```python
from build123d import *

# Parameters (mm, degrees)
SKETCH1_R           = 1.8
SKETCH1_W           = 13
SKETCH1_H           = 7.25
BOSS_EXTRUDE1_DEPTH = 1
SKETCH2_R           = 3
SKETCH2_R_2         = 1.8
BOSS_EXTRUDE2_DEPTH = 5.8
FILLET4_R           = 2
FILLET5_R           = 2
FILLET6_R           = 2
FILLET7_R           = 2


with BuildPart() as part:
    # Sketch1 → Boss-Extrude1 (new body)
    with BuildSketch(Plane.XY):
        with BuildLine():
            Line((-6.5, 11), (6.5, 11))
            Line((6.5, 11), (10.25, 11))
            Line((10.25, 11), (10.25, 3))
            ThreePointArc((10.25, 3), (13.25, 0), (10.25, -3))
            Line((10.25, -3), (10.25, -11))
            Line((10.25, -11), (6.5, -11))
            Line((6.5, -11), (-6.5, -11))
            Line((-6.5, -11), (-10.25, -11))
            Line((-10.25, -11), (-10.25, -3))
            ThreePointArc((-10.25, -3), (-13.25, 0), (-10.25, 3))
            Line((-10.25, 3), (-10.25, 11))
            Line((-10.25, 11), (-6.5, 11))
        make_face()
        with Locations(Location((-10.25, 0, 0), (0, 0, 180))):
            Circle(SKETCH1_R, mode=Mode.SUBTRACT)
        with Locations((10.25, 0)):
            Circle(SKETCH1_R, mode=Mode.SUBTRACT)
        with Locations((0, -4.875)):
            Rectangle(SKETCH1_W, SKETCH1_H, mode=Mode.SUBTRACT)
        with Locations((0, 4.875)):
            Rectangle(SKETCH1_W, SKETCH1_H, mode=Mode.SUBTRACT)
    extrude(amount=BOSS_EXTRUDE1_DEPTH)

    # Sketch2 → Boss-Extrude2 (add)
    with BuildSketch(Plane.XY.offset(1)):
        with Locations(Location((-10.25, 0, 0), (0, 0, 270))):
            Circle(SKETCH2_R)
        with Locations(Location((-10.25, 0, 0), (0, 0, 180))):
            Circle(SKETCH2_R_2, mode=Mode.SUBTRACT)
        with Locations(Location((10.25, 0, 0), (0, 0, 180))):
            Circle(SKETCH2_R)
        with Locations(Location((10.25, 0, 0), (0, 0, 180))):
            Circle(SKETCH2_R_2, mode=Mode.SUBTRACT)
    extrude(amount=BOSS_EXTRUDE2_DEPTH)

    # Fillet4
    fillet4_edges = [part.edges().sort_by_distance(p)[0] for p in [
        (-10.25, 11, 0.5),
    ]]
    fillet(fillet4_edges, radius=FILLET4_R)

    # Fillet5
    fillet5_edges = [part.edges().sort_by_distance(p)[0] for p in [
        (10.25, 11, 0.5),
    ]]
    fillet(fillet5_edges, radius=FILLET5_R)

    # Fillet6
    fillet6_edges = [part.edges().sort_by_distance(p)[0] for p in [
        (-10.25, -11, 0.5),
    ]]
    fillet(fillet6_edges, radius=FILLET6_R)

    # Fillet7
    fillet7_edges = [part.edges().sort_by_distance(p)[0] for p in [
        (10.25, -11, 0.5),
    ]]
    fillet(fillet7_edges, radius=FILLET7_R)


solid = part.part
```
Can you work these out from the model? Positions are in its coordinate system, mm. A direction names the side the tool comes from. Give positions to 0.01 mm unless a question says otherwise; leave off trailing zeros. Loops run counter-clockwise (first coordinate to the right, second up) from the corner with the lowest first, then second, coordinate; pieces in that order, holes last. Notation, with made-up numbers: M -30,-18.75 L 0,-18.75 A21 ccw 0,0.25 Z; hole C 46,-3.75 d3. An arc over 180 degrees is marked long. Answer in a Markdown table with one row per item.
1. Suppose I cut it at B-B on x = -5.25. Write out the boundary of the cut face in (y, z).
Taken from the geometry:
| item | result |
|---|---|
| outline | M -11,0 L -8.5,0 L -8.5,1 L -11,1 Z; M -1.25,0 L 1.25,0 L 1.25,1 L -1.25,1 Z; M 8.5,0 L 11,0 L 11,1 L 8.5,1 Z |
2. For pin 1 Ø10 at (x, y) = (-3, -7) entering from +Z; pin 2 Ø1.1 at (y, z) = (6, 0.5) entering from +X; pin 3 Ø0.5 at (y, z) = (-5, 0.5) entering from -X; pin 4 Ø4 at (x, y) = (10.25, 0) entering from -Z, each with a flat end and sliding along its axis, tell me the tip position at first contact or that it passes through.
Taken from the geometry:
| item | result |
|---|---|
| pin 1 | stops at z = 1 |
| pin 2 | stops at x = 10.25 |
| pin 3 | stops at x = -10.25 |
| pin 4 | stops at z = 0 |
3. If I drill on line 1 along Y through (x, z) = (-2, 0.75); line 2 along Y through (x, z) = (10.25, 4.55); line 3 along X through (y, z) = (-0.5, 4.25), over which ranges is the centre line in solid material (lowest first)?
Taken from the geometry:
| item | result |
|---|---|
| line 1 | y = -11 to -8.5, -1.25 to 1.25, 8.5 to 11 |
| line 2 | y = -3 to -1.8, 1.8 to 3 |
| line 3 | x = -13.21 to -11.98, -8.52 to -7.29, 7.29 to 8.52, 11.98 to 13.21 |
4. Which directions (+Z, -Z, +X, -X, +Y, -Y) give clear straight access to the entire face, cutting with the end or side of a thin tool? Please do faces 4 (the flat face through (10.25, -6, 0.5)), 5 (the flat face through (-6.5, 4.8, 0.5)), 6 (the flat face through (0, 0, 1)).
Taken from the geometry:
| item | result |
|---|---|
| face 4 | +Z, -Z, +X, -Y |
| face 5 | +Z, -Z |
| face 6 | +Z |
5. Suppose I cut it at C-C on y = 4. Write out the boundary of the cut face in (x, z).
Taken from the geometry:
| item | result |
|---|---|
| outline | M -10.25,0 L -6.5,0 L -6.5,1 L -10.25,1 Z; M 6.5,0 L 10.25,0 L 10.25,1 L 6.5,1 Z |
6. Suppose I cut it at A-A on y = 0. Write out the boundary of the cut face in (x, z).
Taken from the geometry:
| item | result |
|---|---|
| outline | M -13.25,0 L -12.05,0 L -12.05,6.8 L -13.25,6.8 Z; M -8.45,0 L 8.45,0 L 8.45,6.8 L 7.25,6.8 L 7.25,1 L -7.25,1 L -7.25,6.8 L -8.45,6.8 Z; M 12.05,0 L 13.25,0 L 13.25,6.8 L 12.05,6.8 Z |
7. Thinking about a two-plate mould opening in X: for faces 1 (the cylindrical face through (9.65, -10.43, 0.51)), 2 (the flat face through (0, 0, 0)), 3 (the flat face through (-0.1, -1.25, 0.5)), which applies, released by +X, released by -X, zero draft, split by the parting line, or undercut?
Taken from the geometry:
| item | result |
|---|---|
| face 1 | released by +X |
| face 2 | zero draft |
| face 3 | undercut |
8. Suppose I cut it at D-D on z = 0.5. Write out the boundary of the cut face in (x, y).
Taken from the geometry:
| item | result |
|---|---|
| outline | M -10.25,-9 A2 ccw -8.25,-11 L 8.25,-11 A2 ccw 10.25,-9 L 10.25,-3 A3 ccw 10.25,3 L 10.25,9 A2 ccw 8.25,11 L -8.25,11 A2 ccw -10.25,9 L -10.25,3 A3 ccw -10.25,-3 Z; hole C -10.25,0 d3.6; hole M -6.5,-8.5 L 6.5,-8.5 L 6.5,-1.25 L -6.5,-1.25 Z; hole M -6.5,1.25 L 6.5,1.25 L 6.5,8.5 L -6.5,8.5 Z; hole C 10.25,0 d3.6 |
